```python
from build123d import *

# Parameters (mm, degrees)
SKETCH1_R                = 48.5
SKETCH1_R_2              = 1.5
SKETCH1_R_3              = 2.235591035
BOSS_EXTRUDE2_DEPTH      = 4
BOSS_EXTRUDE3_DEPTH      = 0.0001
BOSS_EXTRUDE3_DEPTH_BACK = 14
SKETCH6_R                = 10
CUT_EXTRUDE1_DEPTH       = 12
SKETCH11_R               = 1.3
CUT_EXTRUDE3_DEPTH       = 4
CUT_EXTRUDE4_DEPTH       = 2
CUT_EXTRUDE5_DEPTH       = 2


with BuildPart() as part:
    # Sketch1 → Boss-Extrude2 (new body)
    with BuildSketch(Plane(origin=(0, 0, 0), x_dir=(1, 0, 0), z_dir=(0, 1, 0))):
        with Locations(Location((0, 0, 0), (0, 0, 270))):
            Circle(SKETCH1_R)
        with Locations(Location((0, 7.25, 0), (0, 0, 270))):
            Circle(SKETCH1_R_2, mode=Mode.SUBTRACT)
        with Locations(Location((0, -7.25, 0), (0, 0, 270))):
            Circle(SKETCH1_R_2, mode=Mode.SUBTRACT)
        with Locations(Location((0, 0, 0), (0, 0, 270))):
            Circle(SKETCH1_R_3, mode=Mode.SUBTRACT)
    extrude(amount=BOSS_EXTRUDE2_DEPTH)

    # Sketch6 → Boss-Extrude3 (add, two sides: drawn at the far end of the back side and taken through both)
    with BuildSketch(Plane(origin=(-5, 0, 0), x_dir=(0, 0, -1), z_dir=(1, 0, 0)).offset(-BOSS_EXTRUDE3_DEPTH_BACK)):
        with BuildLine():
            Line((25.18, 4), (-35.5, 4))
            Line((-35.5, 4), (-35.5, 12.01726107))
            ThreePointArc((-35.5, 12.01726107), (-34.084736696, 21.902425823), (-29.952654999, 30.993374798))
            Line((-29.952654999, 30.993374798), (-14.438105641, 55.261411059))
            ThreePointArc((-14.438105641, 55.261411059), (25.491097233, 62.28169582), (29.092718415, 21.900339167))
            ThreePointArc((29.092718415, 21.900339167), (26.192340729, 17.214399439), (25.18, 11.79726107))
            Line((25.18, 11.79726107), (25.18, 4))
        make_face()
        with Locations((8.75, 40.43726107)):
            Circle(SKETCH6_R, mode=Mode.SUBTRACT)
    extrude(amount=BOSS_EXTRUDE3_DEPTH + BOSS_EXTRUDE3_DEPTH_BACK)

    # Sketch9 → Cut-Extrude1 (cut)
    with BuildSketch(Plane.ZY.offset(19)):
        Polygon((5.568912319, 11.269106346), (20.418154724, 26.118348751), (-8.573223305, 55.109726779), (-23.42246571, 40.260484374), align=None)
    extrude(amount=-CUT_EXTRUDE1_DEPTH, mode=Mode.SUBTRACT)

    # Sketch11 → Cut-Extrude3 (cut)
    with BuildSketch(Plane.ZY.offset(19)):
        with Locations((-15.14931637, 53.907645251)):
            Circle(SKETCH11_R)
        with Locations(Location((-22.220384182, 46.836577439, 0), (0, 0, 180))):
            Circle(SKETCH11_R)
        with Locations((12.145005384, 12.471187874)):
            Circle(SKETCH11_R)
        with Locations(Location((19.216073196, 19.542255686, 0), (0, 0, 180))):
            Circle(SKETCH11_R)
    extrude(amount=-CUT_EXTRUDE3_DEPTH, mode=Mode.SUBTRACT)

    # Sketch16 → Cut-Extrude4 (cut)
    with BuildSketch(Plane.ZY.offset(19)):
        with BuildLine():
            Line((-16.875075084, 4), (28.737520082, 4))
            add(Edge.make_bspline(
                [(-16.875075084, 4), (-17.737013272, 15.160077135), (-34.124977495, 25.159288994), (-33.933000746, 51.000691554), (-17.215111481, 67.555057226), (7.98292021, 62.524626035), (20.715664688, 35.805630134), (37.029137104, 21.254502483), (28.737520082, 4)],
                knots=[0, 0, 0, 0, 0.199147198, 0.31666239, 0.448197293, 0.600919397, 0.725180292, 1, 1, 1, 1], degree=3))
        make_face()
    extrude(amount=-CUT_EXTRUDE4_DEPTH, mode=Mode.SUBTRACT)

    # Sketch18 → Cut-Extrude5 (cut)
    with BuildSketch(Plane.ZY.offset(7)):
        with BuildLine():
            Line((11.727812383, 19.959448687), (8.856958852, 22.830302218))
            Line((8.856958852, 22.830302218), (5.98610532, 19.959448687))
            ThreePointArc((5.98610532, 19.959448687), (8.856958852, 18.770302218), (11.727812383, 19.959448687))
        make_face()
        with BuildLine():
            Line((11.727812383, 25.70115575), (8.856958852, 22.830302218))
            Line((8.856958852, 22.830302218), (11.727812383, 19.959448687))
            ThreePointArc((11.727812383, 19.959448687), (12.916958852, 22.830302218), (11.727812383, 25.70115575))
        make_face()
        with BuildLine():
            ThreePointArc((1.25, 40.43726107), (0.488795325, 36.610426746), (-1.678932188, 33.366193258))
            Line((-1.678932188, 33.366193258), (8.856958852, 22.830302218))
            Line((8.856958852, 22.830302218), (11.727812383, 25.70115575))
            Line((11.727812383, 25.70115575), (15.220919882, 29.194263249))
            Line((15.220919882, 29.194263249), (0.696168032, 43.719015099))
            ThreePointArc((0.696168032, 43.719015099), (1.110569971, 42.101340346), (1.25, 40.43726107))
        make_face()
        with BuildLine():
            Line((8.856958852, 22.830302218), (-1.678932188, 33.366193258))
            ThreePointArc((-1.678932188, 33.366193258), (-6.513932022, 30.690466725), (-12.031754029, 30.991093038))
            Line((-12.031754029, 30.991093038), (2.492997821, 16.466341187))
            Line((2.492997821, 16.466341187), (5.98610532, 19.959448687))
            Line((5.98610532, 19.959448687), (8.856958852, 22.830302218))
        make_face()
    extrude(amount=-CUT_EXTRUDE5_DEPTH, mode=Mode.SUBTRACT)


solid = part.part
```
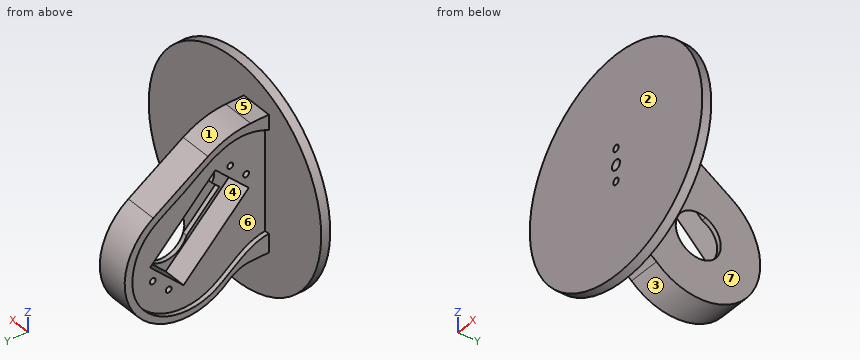
Here's how the part is built. I have some questions about the finished solid (model axes, mm). Face numbers are marked on the shaded views. A direction names the side the tool comes from. Round coordinates to 2 decimals unless told otherwise and drop trailing zeros. Order: outer loops, then holes, each group sorted by start corner. A loop starts at its lowest first (then second) coordinate and runs counter-clockwise, first axis right, second up. Notation, with made-up numbers: M 4.5,-16.75 L 13.5,-16.75 A3 cw 13.5,-11.75 Z; hole C 49.5,-31 d3. An arc over 180 degrees is marked long. Answer in a Markdown table with one row per item.
Item 1: Thinking about a two-plate mould opening in Y: for the marked faces 1, 2, 3 and 4, which applies, +Y half, -Y half, draft (parallel to the pull), parting line (faces both ways), or undercut?
A:
| item | result |
|---|---|
| face 1 | +Y half |
| face 2 | -Y half |
| face 3 | undercut |
| face 4 | undercut |
Item 2: Imagine slicing it at A-A, the plane x = 0. Write out the boundary of the cut face in (y, z), and give its area (3 significant figures).
A:
| item | result |
|---|---|
| outline | M 0,-48.5 L 4,-48.5 L 4,-8.75 L 0,-8.75 Z; M 0,-5.75 L 4,-5.75 L 4,-2.24 L 0,-2.24 Z; M 0,2.24 L 4,2.24 L 4,5.75 L 0,5.75 Z; M 0,8.75 L 4,8.75 L 4,48.5 L 0,48.5 Z |
| area | 346 mm2 |
Item 3: For the marked faces 5, 6 and 7, which set-ups out of +Z, -Z, +X, -X, +Y, -Y let a thin tool reach every point of the face, with its end or its side?
A:
| item | result |
|---|---|
| face 5 | +Z, +X, -X, +Y |
| face 6 | -X |
| face 7 | +Z, -Z, +X, +Y |
Item 4: I'm going to push flat-ended pins straight in: pin 1 (2.5 mm diameter, centred on x = -10.5, y = 6, fed in from -Z); pin 2 (4 mm diameter, centred on y = 20, z = -18.5, fed in from +X); pin 3 (2 mm diameter, centred on y = 46.84, z = -22.22, fed in from -X). Where does each tip first touch, or does it pass through?
A:
| item | result |
|---|---|
| pin 1 | stops at z = -25.18 |
| pin 2 | stops at x = -5 |
| pin 3 | stops at x = -15 |
Item 5: If I drill on L1, parallel to Y at x = -33.5, z = 28; L2, parallel to X at y = 8, z = 11; L3, parallel to Y at x = -6.05, z = -8.75, over which ranges is the centre line in solid material (lowest first)? Write a range as from..to.
A:
| item | result |
|---|---|
| L1 | y = 0..4 |
| L2 | x = -17..-5 |
| L3 | y = 0..27.71, 50.44..67.96 |
Item 6: Imagine slicing it at B-B, the plane z = -41. Write out the boundary of the cut face in (x, y).
A:
| item | result |
|---|---|
| outline | M -25.91,0 L 25.91,0 L 25.91,4 L -25.91,4 Z |
Item 7: Imagine slicing it at C-C, the plane x = -22.5. Write out the boundary of the cut face in (y, z), and give its area (3 significant figures).
A:
| item | result |
|---|---|
| outline | M 0,-42.97 L 4,-42.97 L 4,42.97 L 0,42.97 Z |
| area | 344 mm2 |
